The model under review builds one solid part; all positions refer to its coordinate system, in mm. A direction names the side the tool comes from. Give positions to 0.01 mm unless a question says otherwise; leave off trailing zeros. Write each loop counter-clockwise with the first axis right and the second up, starting at its lowest first coordinate (ties: lowest second). Pieces come first, ordered by that corner, then holes. Notation, with made-up numbers: M -11.5,85 L 4.5,85 A29 ccw 4.5,113 Z; hole C -9,62.25 d4. An arc over 180 degrees is marked long. Write item = value, one per line. Start each with the question number.
```python
from build123d import *
from OCP.BRepFilletAPI import BRepFilletAPI_MakeChamfer

# Parameters (mm, degrees)
CUT_EXTRUDE1_START = -7.5
CUT_EXTRUDE1_DEPTH = 7.5
CUT_EXTRUDE3_START = -60
CUT_EXTRUDE3_DEPTH = 60
CUT_EXTRUDE4_DEPTH = 9
CHAMFER1_SIZE      = 1
CHAMFER1_SIZE2     = 0.730484553


with BuildPart() as part:
    # Sketch1 → Revolve1 (revolve)
    with BuildSketch(Plane.XY, mode=Mode.PRIVATE) as revolve1_sk:
        Polygon((4, 0), (10, 0), (10, -4), (8.25, -5.75), (8.25, -77.5), (4, -80), align=None)
    revolve(revolve1_sk.sketch.rotate(Axis((0, 0, 0), (0, -1, 0)), 90), axis=Axis((0, 0, 0), (0, -1, 0)))

    # Sketch3 → Cut-Extrude1 (cut)
    with BuildSketch(Plane(origin=(0, -8.75, 0), x_dir=(1, 0, 0), z_dir=(0, 1, 0)).offset(CUT_EXTRUDE1_START)):
        with BuildLine():
            ThreePointArc((4.242640687, 4.242640687), (0, 6), (-4.242640687, 4.242640687))
            Line((-4.242640687, 4.242640687), (-6.363961031, 2.121320344))
            Line((-6.363961031, 2.121320344), (-7.555586623, 3.312945936))
            ThreePointArc((-7.555586623, 3.312945936), (0, 8.25), (7.555586623, 3.312945936))
            Line((7.555586623, 3.312945936), (6.363961031, 2.121320344))
            Line((6.363961031, 2.121320344), (4.242640687, 4.242640687))
        make_face()
        with BuildLine():
            ThreePointArc((7.555586623, -3.312945936), (0, -8.25), (-7.555586623, -3.312945936))
            Line((-7.555586623, -3.312945936), (-6.363961031, -2.121320344))
            Line((-6.363961031, -2.121320344), (-4.242640687, -4.242640687))
            ThreePointArc((-4.242640687, -4.242640687), (0, -6), (4.242640687, -4.242640687))
            Line((4.242640687, -4.242640687), (6.363961031, -2.121320344))
            Line((6.363961031, -2.121320344), (7.555586623, -3.312945936))
        make_face()
    extrude(amount=CUT_EXTRUDE1_DEPTH, mode=Mode.SUBTRACT)

    # Sketch4 → Cut-Extrude3 (cut)
    with BuildSketch(Plane(origin=(0, -16.25, 0), x_dir=(1, 0, 0), z_dir=(0, 1, 0)).offset(CUT_EXTRUDE3_START)):
        with BuildLine():
            Line((2.807762918, 7.757510386), (1.767766953, 6.717514421))
            Line((1.767766953, 6.717514421), (6.363961031, 2.121320344))
            Line((6.363961031, 2.121320344), (7.555586623, 3.312945936))
            ThreePointArc((7.555586623, 3.312945936), (5.638110651, 6.022807342), (2.807762918, 7.757510386))
        make_face()
        with BuildLine():
            Line((-7.555586623, 3.312945936), (-6.363961031, 2.121320344))
            Line((-6.363961031, 2.121320344), (-1.767766953, 6.717514421))
            Line((-1.767766953, 6.717514421), (-2.807762918, 7.757510386))
            ThreePointArc((-2.807762918, 7.757510386), (-5.638110651, 6.022807342), (-7.555586623, 3.312945936))
        make_face()
        with BuildLine():
            Line((-1.767766953, -6.717514421), (-2.807762918, -7.757510386))
            ThreePointArc((-2.807762918, -7.757510386), (-5.638110651, -6.022807342), (-7.555586623, -3.312945936))
            Line((-7.555586623, -3.312945936), (-6.363961031, -2.121320344))
            Line((-6.363961031, -2.121320344), (-1.767766953, -6.717514421))
        make_face()
        with BuildLine():
            Line((7.555586623, -3.312945936), (6.363961031, -2.121320344))
            Line((6.363961031, -2.121320344), (1.767766953, -6.717514421))
            Line((1.767766953, -6.717514421), (2.807762918, -7.757510386))
            ThreePointArc((2.807762918, -7.757510386), (5.638110651, -6.022807342), (7.555586623, -3.312945936))
        make_face()
    extrude(amount=CUT_EXTRUDE3_DEPTH, mode=Mode.SUBTRACT)

    # Sketch6 → Cut-Extrude4 (cut)
    with BuildSketch(Plane(origin=(0, -76.25, 0), x_dir=(1, 0, 0), z_dir=(0, 1, 0))):
        with BuildLine():
            Line((2.807762918, -7.757510386), (1.767766953, -6.717514421))
            Line((1.767766953, -6.717514421), (4.065863992, -4.419417382))
            ThreePointArc((4.065863992, -4.419417382), (6.005206075, 0), (4.065863992, 4.419417382))
            Line((4.065863992, 4.419417382), (1.767766953, 6.717514421))
            Line((1.767766953, 6.717514421), (2.807762918, 7.757510386))
            ThreePointArc((2.807762918, 7.757510386), (8.25, 0), (2.807762918, -7.757510386))
        make_face()
        with BuildLine():
            Line((-1.767766953, 6.717514421), (-2.807762918, 7.757510386))
            ThreePointArc((-2.807762918, 7.757510386), (-8.25, 0), (-2.807762918, -7.757510386))
            Line((-2.807762918, -7.757510386), (-1.767766953, -6.717514421))
            Line((-1.767766953, -6.717514421), (-4.065863992, -4.419417382))
            ThreePointArc((-4.065863992, -4.419417382), (-6.005206075, 0), (-4.065863992, 4.419417382))
            Line((-4.065863992, 4.419417382), (-1.767766953, 6.717514421))
        make_face()
    extrude(amount=CUT_EXTRUDE4_DEPTH, mode=Mode.SUBTRACT)

    # Chamfer1: one chamfer whose edges measure the first distance from different faces: ONE call of the kernel's chamfer builder (chamfer() names one face for all edges)
    chamfer1_edges_1 = [part.edges().sort_by_distance(p)[0] for p in [
        (0, 0, -4),
    ]]
    chamfer1_edges_2 = [part.edges().sort_by_distance(p)[0] for p in [
        (0, -80, -4),
    ]]
    chamfer1_side_2 = [part.faces().sort_by_distance(p)[0] for p in [
        (0, -40, -4),
    ]]
    chamfer1 = BRepFilletAPI_MakeChamfer(part.part.solid().wrapped)
    for e in chamfer1_edges_1:
        chamfer1.Add(CHAMFER1_SIZE, e.wrapped)
    for e in chamfer1_edges_2:
        chamfer1.Add(CHAMFER1_SIZE, CHAMFER1_SIZE2, e.wrapped, chamfer1_side_2[0].wrapped)  # the first distance lies on this face
    add(Compound.cast(chamfer1.Shape()), mode=Mode.REPLACE)


solid = part.part
```
Item 1: For faces 4 (the flat face through (6.5, -76.25, -0.1)), 5 (the cylindrical face through (0, -13, 6)), 6 (the cylindrical face through (-2.02, -51.55, -8)), 7 (the cylindrical face through (0, -13, -6)), list the 3-axis set-ups (+Z, -Z, +X, -X, +Y, -Y) from which the entire face can be reached by the end or side of a thin tool; tool diameter is ignored.
Item 2: We need section A-A, the plane y = -48.5. Write out the cut boundary in (x, z).
Item 3: To check wall thickness, follow probe 1 along X at (y, z) = (-20, 2.5); probe 2 along X at (y, z) = (-46.5, 0); probe 3 along X at (y, z) = (-75, -0.5). State the ranges of each line that lie inside material, in increasing order. Write a range as [from, to].
Item 4: The part is to be moulded in two halves that separate along Y. For faces 1 (the cylindrical face through (0, -2, -10)), 2 (the flat face through (0, -8.75, 7)), 3 (the conical face through (4.263, -79.526, 2.217)), say which applies: released by +Y, released by -Y, zero draft, split by the parting line, or undercut.
Item 5: Clearance check with flat-ended pins moving along their axes: P1, Ø1, axis at x = -6, y = -40.5, coming from the +Z side; P2, Ø5, axis at x = 0, z = -4, coming from the -Y side; P3, Ø1.5, axis at y = -62.5, z = -1.5, coming from the -X side; P4, Ø3, axis at x = -5.5, y = -37, coming from the +Z side. State where each tip first meets the part, or that it passes through.
Worked out:
q1.face_4 = +X
q1.face_5 = +Z
q1.face_6 = -Y
q1.face_7 = -Z
q2.outline = M -7.56,-3.31 L -6.36,-2.12 L -1.77,-6.72 L -2.81,-7.76 A8.25 ccw 2.81,-7.76 L 1.77,-6.72 L 6.36,-2.12 L 7.56,-3.31 A8.25 ccw 7.56,3.31 L 6.36,2.12 L 1.77,6.72 L 2.81,7.76 A8.25 ccw -2.81,7.76 L -1.77,6.72 L -6.36,2.12 L -7.56,3.31 A8.25 ccw Z; hole C 0,0 d8
q3.probe_1 = [-7.86, -6.74], [-5.99, -3.12], [3.12, 5.99], [6.74, 7.86]
q3.probe_2 = [-8.25, -4], [4, 8.25]
q3.probe_3 = [-5.98, -3.97], [3.97, 5.98]
q4.face_1 = zero draft
q4.face_2 = undercut
q4.face_3 = released by -Y
q5.P1 = 2.99
q5.P2 = -79.63
q5.P3 = -8.22
q5.P4 = 4.49
